from build123d import *

# Parameters (mm, degrees)
SKETCH_1_R          = 5
EXTRUDE_1_DEPTH     = 20
SKETCH_2_R          = 15
SKETCH_2_R_2        = 10
EXTRUDE_2_DEPTH     = 50
SKETCH_3_W          = 53.583106362
SKETCH_3_H          = 4
CUT_EXTRUDE_1_DEPTH = 10


with BuildPart() as part:
    # 草圖1 → 填料-伸長1 (new body)
    with BuildSketch(Plane.XY):
        with BuildLine():
            ThreePointArc((-30.980762114, -6.339745962), (-34.641016151, -20), (-20.980762114, -23.660254038))
            Line((-20.980762114, -23.660254038), (-10, -17.320508076))
            ThreePointArc((-10, -17.320508076), (0, -20), (10, -17.320508076))
            Line((10, -17.320508076), (20.980762114, -23.660254038))
            ThreePointArc((20.980762114, -23.660254038), (34.641016151, -20), (30.980762114, -6.339745962))
            Line((30.980762114, -6.339745962), (20, 0))
            ThreePointArc((20, 0), (17.320508076, 10), (10, 17.320508076))
            Line((10, 17.320508076), (10, 30))
            ThreePointArc((10, 30), (0, 40), (-10, 30))
            Line((-10, 30), (-10, 17.320508076))
            ThreePointArc((-10, 17.320508076), (-17.320508076, 10), (-20, 0))
            Line((-20, 0), (-30.980762114, -6.339745962))
        make_face()
        with Locations((-25.980762114, -15)):
            Circle(SKETCH_1_R, mode=Mode.SUBTRACT)
        with Locations((25.980762114, -15)):
            Circle(SKETCH_1_R, mode=Mode.SUBTRACT)
        with Locations((0, 30)):
            Circle(SKETCH_1_R, mode=Mode.SUBTRACT)
    extrude(amount=EXTRUDE_1_DEPTH)

    # 草圖2 → 填料-伸長2 (add)
    with BuildSketch(Plane.XY.offset(20)):
        Circle(SKETCH_2_R)
        Circle(SKETCH_2_R_2, mode=Mode.SUBTRACT)
    extrude(amount=EXTRUDE_2_DEPTH)

    # 草圖3 → 除料-伸長1 (cut)
    with BuildSketch(Plane.XY.offset(70)):
        Rectangle(SKETCH_3_W, SKETCH_3_H)
    extrude(amount=-CUT_EXTRUDE_1_DEPTH, mode=Mode.SUBTRACT)


solid = part.part
Geometry check sheet. Reference: the model listing, model coordinates, mm. A direction names the side the tool comes from. Give positions to 0.01 mm unless a question says otherwise; leave off trailing zeros. Loops run counter-clockwise (first coordinate to the right, second up) from the corner with the lowest first, then second, coordinate; pieces in that order, holes last. Notation, with made-up numbers: M -34.75,74.25 L -30.75,74.25 A15 cw -30.75,102.25 Z; hole C -14.75,48 d6. An arc over 180 degrees is marked long. Write each question's results on one line, items separated by ' | '.
1) Section check D-D, the plane x = 30. Record the boundary of the cut face in (y, z), plus the area to 3 significant figures.
Answers follow:
outline: M -24.16,0 L -17.97,0 L -17.97,20 L -24.16,20 Z; M -12.03,0 L -5.77,0 L -5.77,20 L -12.03,20 Z | area: 249 mm2
2) Thickness scan on line 1 (X direction, y = 0, z = 49.5); line 2 (Z direction, x = -8.5, y = 33). Record the ranges inside material, lowest first.
Answers follow:
line 1: -15 to -10, 10 to 15 | line 2: 0 to 20
3) Section check B-B, the plane y = 33. Record the boundary of the cut face in (x, z), plus the area to 3 significant figures.
Answers follow:
outline: M -9.54,0 L -4,0 L -4,20 L -9.54,20 Z; M 4,0 L 9.54,0 L 9.54,20 L 4,20 Z | area: 222 mm2
4) Section check C-C, the plane z = 46. Record the boundary of the cut face in (x, y), plus the area to 3 significant figures.
Answers follow:
outline: C 0,0 d30; hole C 0,0 d20 | area: 393 mm2
5) Release check for a two-part mould opening along Y. For faces 1 (the face through (-17.247, 10.127, 9.86)), 2 (the face through (0, 0, 20)), 3 (the face through (0, 11, 70)) record: +Y half, -Y half, draft (parallel to the pull), parting line (faces both ways), or undercut.
Answers follow:
face 1: +Y half | face 2: undercut | face 3: draft
6) Section check A-A, the plane x = 0. Record the boundary of the cut face in (y, z).
Answers follow:
outline: M -20,0 L 25,0 L 25,20 L 15,20 L 15,70 L 10,70 L 10,20 L -10,20 L -10,70 L -15,70 L -15,20 L -20,20 Z; M 35,0 L 40,0 L 40,20 L 35,20 Z
7) Tool access check on faces 4 (the face through (-8, -14, 20)), 5 (the face through (-10, 24, 10)), 6 (the face through (12, 0, 60)). Record the directions out of +Z, -Z, +X, -X, +Y, -Y that give a thin tool (end or side, any length) a straight path to the whole face; none if there is none.
Answers follow:
face 4: +Z | face 5: +Z, -Z, -X, +Y | face 6: +Z, +X, -X
8) Gauge pin test, flat ends, axial feed: pin 1 (5.5 mm diameter, centred on x = -13, z = 66.5, fed in from +Y); pin 2 (6.5 mm diameter, centred on y = 21.5, z = 10, fed in from +X); pin 3 (8 mm diameter, centred on x = -25.98, y = -15, fed in from +Z); pin 4 (5.5 mm diameter, centred on x = 12.5, z = 65.5, fed in from +Y). Record the tip position at first contact, or that the pin passes through.
Answers follow:
pin 1: y = 10.95 | pin 2: x = 10 | pin 3: through | pin 4: y = 11.4
